from build123d import *

# Parameters (mm, degrees)
SKETCH6_W           = 100
SKETCH6_H           = 100
SKETCH6_R           = 2.1
BOSS_EXTRUDE2_DEPTH = 3
BOSS_EXTRUDE3_DEPTH = 3
SKETCH8_W           = 96
SKETCH8_H           = 2
BOSS_EXTRUDE4_DEPTH = 3
CHAMFER1_SIZE       = 2
BOSS_EXTRUDE5_DEPTH = 3


with BuildPart() as part:
    # Sketch6 → Boss-Extrude2 (new body)
    with BuildSketch(Plane(origin=(0, 0, 0), x_dir=(1, 0, 0), z_dir=(0, 1, 0))):
        with Locations((39.444153985, -113.424821635)):
            Rectangle(SKETCH6_W, SKETCH6_H)
        with Locations((1.68480047, -87.360414745)):
            Circle(SKETCH6_R, mode=Mode.SUBTRACT)
        with Locations((1.68480047, -107.360414745)):
            Circle(SKETCH6_R, mode=Mode.SUBTRACT)
        with Locations((1.68480047, -152.360414745)):
            Circle(SKETCH6_R, mode=Mode.SUBTRACT)
        with Locations((24.444153985, -158.424821635)):
            Circle(SKETCH6_R, mode=Mode.SUBTRACT)
        with Locations((24.444153985, -68.424821635)):
            Circle(SKETCH6_R, mode=Mode.SUBTRACT)
        with Locations((54.444153985, -158.424821635)):
            Circle(SKETCH6_R, mode=Mode.SUBTRACT)
        with Locations((77.2035075, -152.360414745)):
            Circle(SKETCH6_R, mode=Mode.SUBTRACT)
        with Locations((77.2035075, -107.360414745)):
            Circle(SKETCH6_R, mode=Mode.SUBTRACT)
        with Locations((77.2035075, -87.360414745)):
            Circle(SKETCH6_R, mode=Mode.SUBTRACT)
        with Locations((54.444153985, -68.424821635)):
            Circle(SKETCH6_R, mode=Mode.SUBTRACT)
    extrude(amount=BOSS_EXTRUDE2_DEPTH)

    # Sketch7 → Boss-Extrude3 (add)
    with BuildSketch(Plane(origin=(0, 3, 0), x_dir=(1, 0, 0), z_dir=(0, 1, 0))):
        Polygon((-10.555846015, -63.424821635), (-10.555846015, -163.424821635), (-8.555846015, -163.424821635), (-8.555846015, -65.424821635), (87.444153985, -65.424821635), (87.444153985, -163.424821635), (89.444153985, -163.424821635), (89.444153985, -63.424821635), align=None)
    extrude(amount=BOSS_EXTRUDE3_DEPTH)

    # Sketch8 → Boss-Extrude4 (add)
    with BuildSketch(Plane(origin=(0, 3, 0), x_dir=(1, 0, 0), z_dir=(0, 1, 0))):
        with Locations((39.444153985, -162.424821635)):
            Rectangle(SKETCH8_W, SKETCH8_H)
    extrude(amount=BOSS_EXTRUDE4_DEPTH)

    # Chamfer1
    chamfer1_edges = [part.edges().sort_by_distance(p)[0] for p in [
        (-10.555846015, 3, 63.424821635),
        (89.444153985, 3, 63.424821635),
        (89.444153985, 3, 163.424821635),
        (-10.555846015, 3, 163.424821635),
    ]]
    chamfer(chamfer1_edges, length=CHAMFER1_SIZE)

    # Sketch9 → Boss-Extrude5 (add)
    with BuildSketch(Plane(origin=(0, 3, 0), x_dir=(1, 0, 0), z_dir=(0, 1, 0))):
        Polygon((-6.555846015, -65.424821635), (-8.555846015, -67.424821635), (-8.555846015, -65.424821635), align=None)
        Polygon((87.444153985, -67.424821635), (87.444153985, -65.424821635), (85.444153985, -65.424821635), align=None)
        Polygon((85.444153985, -161.424821635), (87.444153985, -159.424821635), (87.444153985, -161.424821635), align=None)
        Polygon((-8.555846015, -159.424821635), (-8.555846015, -161.424821635), (-6.555846015, -161.424821635), align=None)
    extrude(amount=BOSS_EXTRUDE5_DEPTH)


solid = part.part
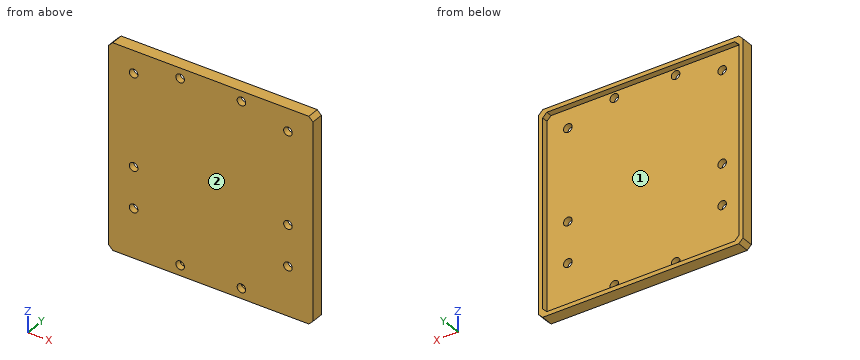
Input: part model. Units: mm. Frame: model coordinates. Face numbers are marked on the shaded views. Round coordinates to 2 decimals unless told otherwise and drop trailing zeros. Loops run counter-clockwise (first coordinate to the right, second up) from the corner with the lowest first, then second, coordinate; pieces in that order, holes last. Notation, with made-up numbers: M -2,68.25 L 3,68.25 A16 cw 3,72.25 Z; hole C 7.25,-34.5 d9. An arc over 180 degrees is marked long. Answer as CSV lines item,"result". Start each with the question number.
(1) Draft query along X for the marked faces 1 and 2. Return one class per face: released by +X, released by -X, zero draft, split by the parting line, or undercut.
(2) Section B-B, the plane x = 18.5. Output: boundary loops of the cut face in (y, z).
(3) Line query: line 1 (Z direction, x = 70, y = 5.3); line 2 (X direction, y = 3.7, z = 79); line 3 (Y direction, x = 0, z = 146). Output: solid intervals per line, ascending. Write a range as [from, to].
(4) Section A-A, the plane y = 4. Output: boundary loops of the cut face in (x, z), plus the area to 3 significant figures.
(5) Section C-C, the plane z = 97. Output: boundary loops of the cut face in (x, y).
(6) First-contact query: pin 1 (5.5 mm diameter, centred on x = 54.44, z = 68.42, fed in from +Y). Flat tip, straight axial feed; report the tip coordinate or a pass-through.
Values found:
1,face 1,"undercut"
1,face 2,"zero draft"
2,outline,"M 0,63.42 L 6,63.42 L 6,65.42 L 3,65.42 L 3,161.42 L 6,161.42 L 6,163.42 L 0,163.42 Z"
3,line 1,"z = [63.42, 65.42], [161.42, 163.42]"
3,line 2,"x = [-10.56, -8.56], [87.44, 89.44]"
3,line 3,"y = [0, 3]"
4,outline,"M -10.56,65.42 L -8.56,63.42 L 87.44,63.42 L 89.44,65.42 L 89.44,161.42 L 87.44,163.42 L -8.56,163.42 L -10.56,161.42 Z; hole M -8.56,67.42 L -6.56,65.42 L 85.44,65.42 L 87.44,67.42 L 87.44,159.42 L 85.44,161.42 L -6.56,161.42 L -8.56,159.42 Z"
4,area,"784 mm²"
5,outline,"M -10.56,0 L 89.44,0 L 89.44,6 L 87.44,6 L 87.44,3 L -8.56,3 L -8.56,6 L -10.56,6 Z"
6,pin 1,"stops at y = 3"
